Here's the drawing with two shaded views (mm, measured from the low corner). I have some questions. A direction names the side the tool comes from. Round coordinates to 2 decimals unless told otherwise and drop trailing zeros. Loops run counter-clockwise (first coordinate to the right, second up) from the corner with the lowest first, then second, coordinate; pieces in that order, holes last.
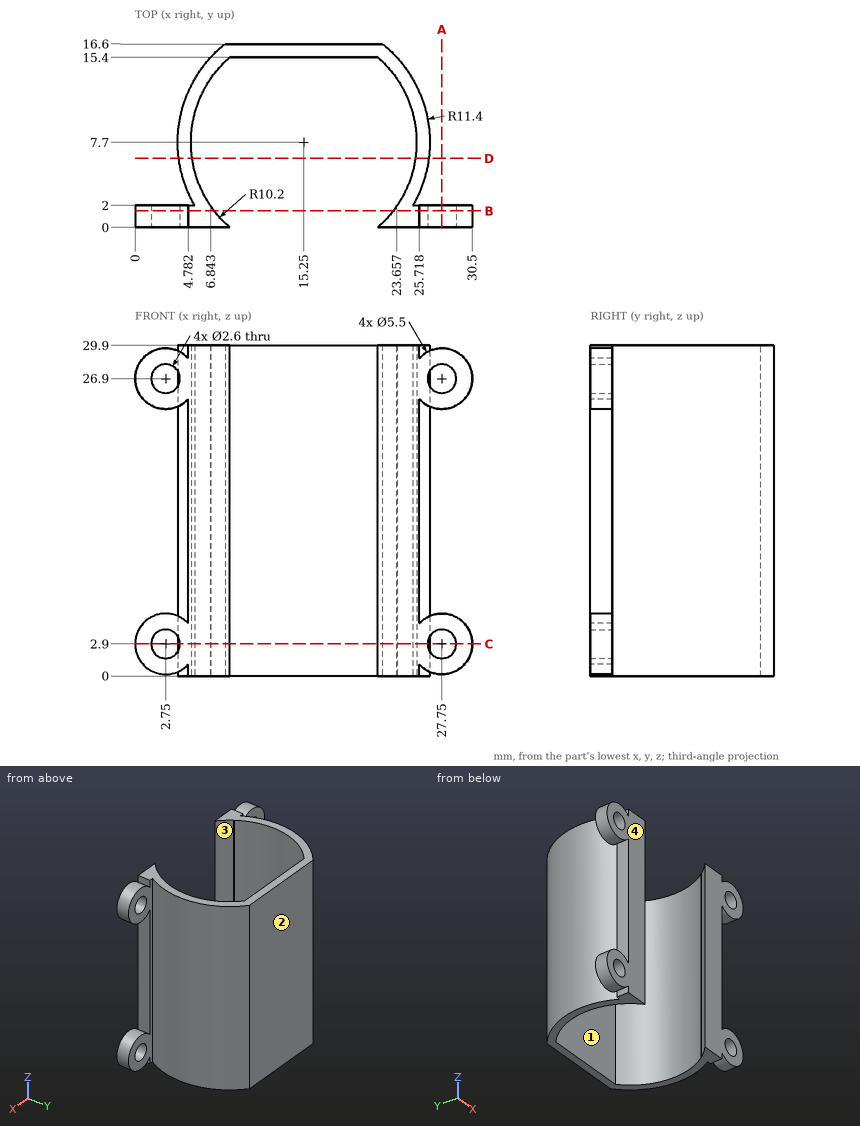
Item 1: If we section it at D-D, the plane y = 6.25: Please give me the cut outline in (x, z).
Results list:
outline: (3.94, 0) - (5.15, 0) - (5.15, 29.9) - (3.94, 29.9) - close; (25.35, 0) - (26.56, 0) - (26.56, 29.9) - (25.35, 29.9) - close
Item 2: We'd pull the mould along X, two halves only. Please class the marked faces 1 and 2: released by +X, released by -X, zero draft, split by the parting line, or undercut.
Results list:
face 1: undercut
face 2: zero draft
Item 3: If we section it at A-A, the plane x = 27.75: Please give me the cut outline in (y, z).
Results list:
outline: (0, 0.15) - (2, 0.15) - (2, 1.6) - (0, 1.6) - close; (0, 4.2) - (2, 4.2) - (2, 5.65) - (0, 5.65) - close; (0, 24.15) - (2, 24.15) - (2, 25.6) - (0, 25.6) - close; (0, 28.2) - (2, 28.2) - (2, 29.65) - (0, 29.65) - close
Item 4: For the marked faces 3 and 4, which set-ups out of +Z, -Z, +X, -X, +Y, -Y let a thin tool reach every point of the face, with its end or its side?
Results list:
face 3: +Z, -Z
face 4: +Z, -Z, +X, -X, -Y
Item 5: If we section it at B-B, the plane y = 1.5: Please give me the cut outline in (x, z).
Results list:
outline: (4.78, 0) - (7.15, 0) - (7.15, 29.9) - (4.78, 29.9) - (4.78, 28.75) arc R2.75 ccw (long way) to (4.78, 25.05) - (4.78, 4.75) arc R2.75 ccw (long way) to (4.78, 1.05) - close; (23.35, 0) - (25.72, 0) - (25.72, 1.05) arc R2.75 ccw (long way) to (25.72, 4.75) - (25.72, 25.05) arc R2.75 ccw (long way) to (25.72, 28.75) - (25.72, 29.9) - (23.35, 29.9) - close; hole circle Ø2.6 at (2.75, 2.9); hole circle Ø2.6 at (2.75, 26.9); hole circle Ø2.6 at (27.75, 2.9); hole circle Ø2.6 at (27.75, 26.9)
Item 6: If I drill on line 1 along X through (y, z) = (7.5, 28); line 2 along Y through (x, z) = (19.5, 17.75); line 3 along X through (y, z) = (6, 16), over which ranges is the centre line in solid material (lowest first)?
Results list:
line 1: x = 3.85 to 5.05, 25.45 to 26.65
line 2: y = 15.4 to 16.6
line 3: x = 3.98 to 5.19, 25.31 to 26.52
Item 7: Will these pins go through, and if not, where does the flat tip stop? pin 1 (0.8 mm diameter, centred on y = 1.5, z = 0.5, fed in from -X); pin 2 (1.6 mm diameter, centred on x = 27.75, z = 26.9, fed in from +Y); pin 3 (3 mm diameter, centred on y = 13, z = 9.5, fed in from +X); pin 4 (2.5 mm diameter, centred on x = 3.5, z = 18, fed in from +Y).
Results list:
pin 1: stops at x = 0.86
pin 2: passes through
pin 3: stops at x = 26
pin 4: stops at y = 12.14
Item 8: If we section it at C-C, the plane z = 2.9: Please give me the cut outline in (x, y).
Results list:
outline: (0, 0) - (1.45, 0) - (1.45, 2) - (0, 2) - close; (4.05, 0) - (8.56, 0) arc R10.2 cw to (6.84, 1.92) - (6.84, 2) - (6.79, 2) arc R10.2 cw to (8.56, 15.4) - (21.94, 15.4) arc R10.2 cw to (23.71, 2) - (23.66, 2) - (23.66, 1.92) arc R10.2 cw to (21.94, 0) - (26.45, 0) - (26.45, 2) - (25.12, 2) arc R11.4 ccw to (22.37, 16.6) - (8.13, 16.6) arc R11.4 ccw to (5.38, 2) - (4.05, 2) - close; (29.05, 0) - (30.5, 0) - (30.5, 2) - (29.05, 2) - close
